from build123d import *

# Parameters (mm, degrees)
PAD_DEPTH       = 1.7
SKETCH009_W     = 14.95
SKETCH009_H     = 14.67
PAD002_DEPTH    = 1.96
SKETCH017_W     = 11.09
SKETCH017_H     = 1.66
POCKET006_DEPTH = 14.6


with BuildPart() as part:
    # Sketch → Pad (new body)
    with BuildSketch(Plane.XY):
        with BuildLine():
            Line((0, 0), (30, 0))
            Line((30, 0), (30, 1))
            Line((30, 1), (31, 1))
            Line((31, 1), (31, 18.27))
            Line((31, 18.27), (24.4, 18.27))
            ThreePointArc((24.4, 24.87), (21.1, 21.57), (24.4, 18.27))
            Line((24.4, 24.87), (31, 24.87))
            Line((31, 24.87), (31, 59.13))
            Line((31, 59.13), (24.4, 59.13))
            ThreePointArc((24.4, 65.73), (21.1, 62.43), (24.4, 59.13))
            Line((24.4, 65.73), (31, 65.73))
            Line((31, 65.73), (31, 83))
            Line((30, 83), (31, 83))
            Line((30, 84), (30, 83))
            Line((30, 84), (0, 84))
            Line((0, 84), (-30, 84))
            Line((-30, 84), (-30, 83))
            Line((-30, 83), (-31, 83))
            Line((-31, 83), (-31, 65.73))
            Line((-31, 65.73), (-24.4, 65.73))
            ThreePointArc((-24.4, 59.13), (-21.1, 62.43), (-24.4, 65.73))
            Line((-24.4, 59.13), (-31, 59.13))
            Line((-31, 59.13), (-31, 24.87))
            Line((-31, 24.87), (-24.4, 24.87))
            ThreePointArc((-24.4, 18.27), (-21.1, 21.57), (-24.4, 24.87))
            Line((-24.4, 18.27), (-31, 18.27))
            Line((-31, 18.27), (-31, 1))
            Line((-31, 1), (-30, 1))
            Line((-30, 1), (-30, 0))
            Line((-30, 0), (0, 0))
        make_face()
    extrude(amount=PAD_DEPTH)

    # Sketch009 → Pad002 (new body)
    with BuildSketch(Plane(origin=(0, 0, 0), x_dir=(1, 0, 0), z_dir=(0, 0, -1))):
        with Locations((22.525, -4.535)):
            Rectangle(SKETCH009_W, SKETCH009_H)
    extrude(amount=PAD002_DEPTH)

    # Sketch017 → Pocket006 (cut)
    with BuildSketch(Plane.XZ.offset(2.8)):
        with Locations((23.575, -0.98)):
            Rectangle(SKETCH017_W, SKETCH017_H)
    extrude(amount=-POCKET006_DEPTH, mode=Mode.SUBTRACT)


solid = part.part
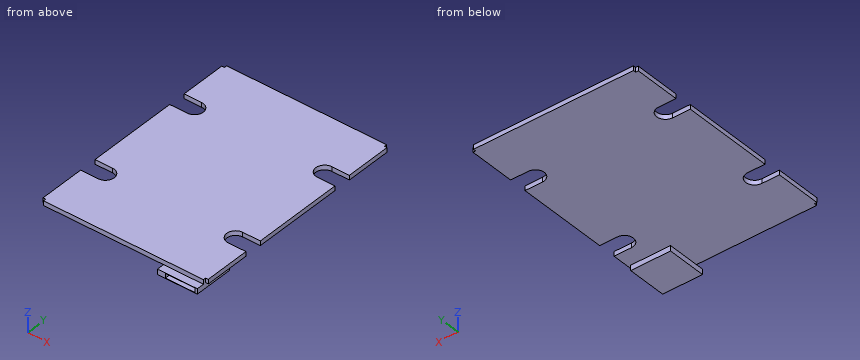
Source: CAD feature listing. Evaluate the final solid. Frame: model axes, mm. Give positions to 0.01 mm unless a question says otherwise; leave off trailing zeros. Write each loop counter-clockwise with the first axis right and the second up, starting at its lowest first coordinate (ties: lowest second). Pieces come first, ordered by that corner, then holes. Notation, with made-up numbers: (11.25, 5) -> (44.25, 5) arc R35 cw to (44.25, 41) -> close; hole circle Ø2 at (-21, -22). An arc over 180 degrees is marked (long way). Write item = value, one per line.
Q1. First-contact query: pin 1 (0.8 mm diameter, centred on y = 3.5, z = -1, fed in from -X); pin 2 (2 mm diameter, centred on y = 35, z = -1.5, fed in from -X); pin 3 (0.8 mm diameter, centred on x = -29, z = 0.5, fed in from -Y); pin 4 (0.5 mm diameter, centred on x = -30.5, z = 1, fed in from +Y). Flat tips, straight axial feed; report the tip coordinate or a pass-through.
Here are the results:
pin_1 = 15.05
pin_2 = through
pin_3 = 0
pin_4 = 83
Q2. Cut plane C-C on y = 21.57. Return loops of the section in (x, z), then the cut area to 3 significant figures.
Here are the results:
outline = (-21.1, 0) -> (21.1, 0) -> (21.1, 1.7) -> (-21.1, 1.7) -> close
area = 71.7 mm²
Q3. Line query: line 1 (Z direction, x = -1.5, y = 1); line 2 (Y direction, x = -15.5, z = 0.8); line 3 (Y direction, x = -24, z = 1.2). Output: solid intervals per line, ascending. Write a range as from..to.
Here are the results:
line_1 = 0..1.7
line_2 = 0..84
line_3 = 0..18.29, 24.85..59.15, 65.71..84
Q4. Cut plane B-B on x = -11. Return loops of the section in (y, z).
Here are the results:
outline = (0, 0) -> (84, 0) -> (84, 1.7) -> (0, 1.7) -> close
Q5. Cut plane A-A on z = 0.75. Return loops of the section in (x, y).
Here are the results:
outline = (-31, 1) -> (-30, 1) -> (-30, 0) -> (30, 0) -> (30, 1) -> (31, 1) -> (31, 18.27) -> (24.4, 18.27) arc R3.3 cw to (24.4, 24.87) -> (31, 24.87) -> (31, 59.13) -> (24.4, 59.13) arc R3.3 cw to (24.4, 65.73) -> (31, 65.73) -> (31, 83) -> (30, 83) -> (30, 84) -> (-30, 84) -> (-30, 83) -> (-31, 83) -> (-31, 65.73) -> (-24.4, 65.73) arc R3.3 cw to (-24.4, 59.13) -> (-31, 59.13) -> (-31, 24.87) -> (-24.4, 24.87) arc R3.3 cw to (-24.4, 18.27) -> (-31, 18.27) -> close
